Could you check a few things on this model? Use its own coordinates, in mm. A direction names the side the tool comes from. Coordinates: 2 decimals unless noted, no trailing zeros. Write each loop counter-clockwise with the first axis right and the second up, starting at its lowest first coordinate (ties: lowest second). Pieces come first, ordered by that corner, then holes.
```python
from build123d import *

# Parameters (mm, degrees)
SKETCH1_R               = 1.6
BOSS_EXTRUDE1_DEPTH     = 8
CUT_EXTRUDE1_DEPTH      = 21.082666196
CUT_EXTRUDE1_DEPTH_BACK = 21.082666196
SKETCH2_R               = 1.75
SKETCH2_R_2             = 1.6


with BuildPart() as part:
    # Sketch1 → Boss-Extrude1 (new body)
    with BuildSketch(Plane(origin=(0, 0, 0), x_dir=(1, 0, 0), z_dir=(0, 1, 0))):
        with BuildLine():
            Line((-6.289674077, 2), (-16.289674077, 2))
            Line((-16.289674077, 2), (-16.289674077, -2))
            Line((-16.289674077, -2), (-6.289674077, -2))
            ThreePointArc((-6.289674077, -2), (0, -6.6), (6.289674077, -2))
            ThreePointArc((6.289674077, -2), (6.6, 0), (6.289674077, 2))
            ThreePointArc((6.289674077, 2), (0, 6.6), (-6.289674077, 2))
        make_face()
        with Locations(Location((0, 0, 0), (0, 0, 270))):
            Circle(SKETCH1_R, mode=Mode.SUBTRACT)
    extrude(amount=BOSS_EXTRUDE1_DEPTH)

    # Sketch2 → Cut-Extrude1 (cut, two sides: drawn at the far end of the back side and taken through both)
    with BuildSketch(Plane.XY.offset(2).offset(-CUT_EXTRUDE1_DEPTH_BACK)):
        with BuildLine():
            Line((-16.289674077, 8), (-16.289674077, 4))
            ThreePointArc((-16.289674077, 4), (-15.118101202, 6.828427125), (-12.289674077, 8))
            Line((-12.289674077, 8), (-16.289674077, 8))
        make_face()
        with BuildLine():
            Line((-16.289674077, 4), (-16.289674077, 0))
            Line((-16.289674077, 0), (-12.289674077, 0))
            ThreePointArc((-12.289674077, 0), (-15.118101202, 1.171572875), (-16.289674077, 4))
        make_face()
        with Locations(Location((-12.289674077, 4, 0), (0, 0, 180))):
            Circle(SKETCH2_R)
        with Locations((0, 4)):
            Circle(SKETCH2_R_2)
    extrude(amount=CUT_EXTRUDE1_DEPTH + CUT_EXTRUDE1_DEPTH_BACK, mode=Mode.SUBTRACT)


solid = part.part
```
1. I want a section at C-C on z = 2.25. Please give me the cut outline in (x, y), plus the area to 3 significant figures.
Verdict:
outline: (-6.2, 0) - (6.2, 0) - (6.2, 8) - (-6.2, 8) - close; hole circle Ø3.2 at (0, 4)
area: 91.2 mm2
2. I want a section at B-B on y = 4.25. Please give me the cut outline in (x, z).
Verdict:
outline: (-16.28, -2) - (-14.02, -2) - (-14.02, 2) - (-16.28, 2) - close; (-10.56, -2) - (-6.29, -2) arc R6.6 ccw to (-1.58, -6.41) - (-1.58, -0.25) arc R1.6 cw to (-1.58, 0.25) - (-1.58, 6.41) arc R6.6 ccw to (-6.29, 2) - (-10.56, 2) - close; (1.58, -6.41) arc R6.6 ccw to (1.58, 6.41) - (1.58, 0.25) arc R1.6 cw to (1.58, -0.25) - close
3. On a 3-axis mill with a long thin cutter (end or side, diameter ignored), from which of +Z, -Z, +X, -X, +Y, -Y can I reach the whole of each face in a straight line? I mean faces 1 (the face through (-10, 4, 2)), 2 (the face through (-1.27, 3.03, 3.99)). Say none if no direction works.
Verdict:
face 1: +Z, -X, +Y, -Y
face 2: +Z, -Z
4. For pin 1 (1 mm diameter, centred on x = -3, y = 1.5, fed in from -Z); pin 2 (1 mm diameter, centred on x = -4.5, y = 2, fed in from +Z); pin 3 (1.5 mm diameter, centred on y = 6, z = -1, fed in from +X); pin 4 (3 mm diameter, centred on x = 0, y = 4, fed in from -Z) (1 decimal), each with a flat end and sliding along its axis, tell me the tip position at first contact or that it passes through.
Verdict:
pin 1: stops at z = -6.11
pin 2: stops at z = 5.25
pin 3: stops at x = 6.6
pin 4: passes through
5. I want a section at D-D on y = 7.25. Please give me the cut outline in (x, z), plus the area to 3 significant figures.
Verdict:
outline: (-14.62, -2) - (-6.29, -2) arc R6.6 ccw (long way) to (-6.29, 2) - (-14.62, 2) - close; hole circle Ø3.2 at (0, 0)
area: 161 mm2
6. Please list where these lines run through material, in increasing order: line 1 along Z through (x, y) = (0, 5.75); line 2 along X through (y, z) = (5.4, 0); line 3 along Z through (x, y) = (-9.5, 5).
Verdict:
line 1: z = -6.6 to -1.6, 1.6 to 6.6
line 2: x = -16.04 to -13.34, -11.24 to -1.6, 1.6 to 6.6
line 3: z = -2 to 2
7. If we mould it in two halves opening along X, with no side actions, what happens to faces 3 (the face through (-1.6, 4.07, -4.08)), 4 (the face through (-10, 4, -2))? For each: pulls with the +X half, pulls with the -X half, needs draft (parallel to the pull), parting line crosses it, or undercut.
Verdict:
face 3: undercut
face 4: needs draft
8. I want a section at A-A on x = 0. Please give me the cut outline in (y, z).
Verdict:
outline: (0, -6.6) - (2.4, -6.6) - (2.4, -1.6) - (0, -1.6) - close; (0, 1.6) - (2.4, 1.6) - (2.4, 6.6) - (0, 6.6) - close; (5.6, -6.6) - (8, -6.6) - (8, -1.6) - (5.6, -1.6) - close; (5.6, 1.6) - (8, 1.6) - (8, 6.6) - (5.6, 6.6) - close
